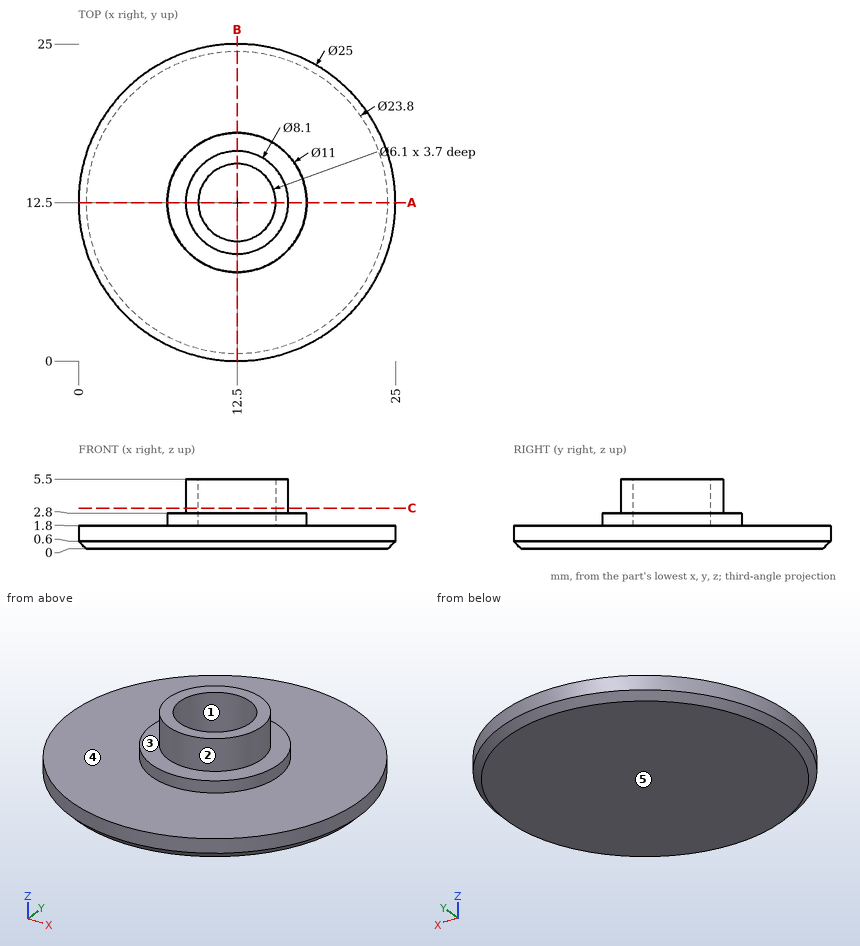
Check sheet for the drawn part. Datum: minimum x, y, z corner. Units: mm. A direction names the side the tool comes from. Coordinates: 2 decimals unless noted, no trailing zeros. Order: outer loops, then holes, each group sorted by start corner. A loop starts at its lowest first (then second) coordinate and runs counter-clockwise, first axis right, second up. Notation, with made-up numbers: M 6.5,29 L 40.5,29 A20 ccw 40.5,37 Z; hole C 56.25,-26.5 d5. An arc over 180 degrees is marked long. One line per item, written item: value. Start each with the question number.
Item 1: Sectioned sample at C-C (z = 3.2). Enter the section's corners in (x, y), then the cut area to 3 significant figures.
Item 2: Mould release check, pull along X, two halves, no side actions. Record for the marked faces 1, 2 and 3: released by +X, released by -X, zero draft, split by the parting line, or undercut.
Item 3: Gauge pin test, flat ends, axial feed: pin 1 (1 mm diameter, centred on x = 22, y = 12.5, fed in from +Z); pin 2 (1 mm diameter, centred on x = 9, z = 4.5, fed in from -Y). Record the tip position at first contact, or that the pin passes through.
Item 4: Sectioned sample at A-A (y = 12.5). Enter the section's corners in (x, z).
Item 5: Access from +Z, -Z, +X, -X, +Y, -Y to the whole of each face (thin tool, end or side, straight path). Record for the marked faces 4 and 5.
Item 6: Scan lines: probe 1 along Y at (x, z) = (12.5, 3.8); probe 2 along Z at (x, y) = (14, 4.75); probe 3 along Z at (x, y) = (7.5, 11.5). Record each from-to range of solid material in increasing order.
Conclusion:
1. outline: C 12.5,12.5 d8.1; hole C 12.5,12.5 d6.1
1. area: 22.3 mm^2
2. face 1: undercut
2. face 2: split by the parting line
2. face 3: zero draft
3. pin 1: stops at z = 1.8
3. pin 2: stops at y = 9.78
4. outline: M 0,0.6 L 0.6,0 L 24.4,0 L 25,0.6 L 25,1.8 L 18,1.8 L 18,2.8 L 16.55,2.8 L 16.55,5.5 L 15.55,5.5 L 15.55,1.8 L 9.45,1.8 L 9.45,5.5 L 8.45,5.5 L 8.45,2.8 L 7,2.8 L 7,1.8 L 0,1.8 Z
5. face 4: +Z
5. face 5: -Z, +X, -X, +Y, -Y
6. probe 1: y = 8.45 to 9.45, 15.55 to 16.55
6. probe 2: z = 0 to 1.8
6. probe 3: z = 0 to 2.8
